Check sheet for the modelled part. Datum: model origin and axes. Units: mm. Face numbers are marked on the shaded views. A direction names the side the tool comes from. Round coordinates to 2 decimals unless told otherwise and drop trailing zeros. Write each loop counter-clockwise with the first axis right and the second up, starting at its lowest first coordinate (ties: lowest second). Pieces come first, ordered by that corner, then holes. Notation, with made-up numbers: (11.5, 57) -> (59.5, 57) arc R7 ccw to (59.5, 70) -> close; hole circle Ø11 at (-37, -0.5). An arc over 180 degrees is marked (long way). One line per item, written item: value.
from build123d import *

# Parameters (mm, degrees)
F0_R     = 1.9
F1_DEPTH = 14.1
F2_DEPTH = 2.1
F3_DEPTH = 10.6
F4_W     = 16.752516
F4_H     = 7.375009
F5_DEPTH = 150
F6_R     = 5
F7_W     = 76.531014
F7_H     = 2.1
F8_DEPTH = 5.5
F9_R     = 1.5


with BuildPart() as f1:
    # F0 (on Top) → F1 (new body)
    with BuildSketch(Plane.XY):
        with BuildLine():
            ThreePointArc((104.3, 0), (101.056497, 1.343503), (102.4, -1.9))
            ThreePointArc((102.4, -1.9), (103.743503, -1.343503), (104.3, 0))
        make_face()
        with BuildLine():
            ThreePointArc((102.4, -23.7), (101.056497, -26.943503), (104.3, -25.6))
            ThreePointArc((104.3, -25.6), (103.743503, -24.256497), (102.4, -23.7))
        make_face()
        with Locations((0, -25.6)):
            Circle(F0_R)
        Circle(F0_R)
    extrude(amount=F1_DEPTH)



with BuildPart() as f2:
    # F0 (on Top) → F2 (new body)
    with BuildSketch(Plane.XY):
        with BuildLine():
            Line((9.95, -14.3), (9.95, -19.3))
            ThreePointArc((9.95, -19.3), (11.414466, -15.764466), (14.95, -14.3))
            Line((14.95, -14.3), (51.2, -14.3))
            Line((51.2, -14.3), (51.2, -11.3))
            Line((51.2, -11.3), (14.95, -11.3))
            ThreePointArc((14.95, -11.3), (11.414466, -9.835534), (9.95, -6.3))
            Line((9.95, -6.3), (9.95, -11.3))
            Line((9.95, -11.3), (9.95, -14.3))
        make_face()
        with BuildLine():
            Line((51.2, -11.3), (51.2, -14.3))
            Line((51.2, -14.3), (67.3, -14.3))
            Line((67.3, -14.3), (72.3, -14.3))
            Line((72.3, -14.3), (87.45, -14.3))
            ThreePointArc((87.45, -14.3), (90.985534, -15.764466), (92.45, -19.3))
            Line((92.45, -19.3), (92.45, -6.3))
            ThreePointArc((92.45, -6.3), (90.985534, -9.835534), (87.45, -11.3))
            Line((87.45, -11.3), (72.3, -11.3))
            Line((72.3, -11.3), (67.3, -11.3))
            Line((67.3, -11.3), (51.2, -11.3))
        make_face()
    extrude(amount=F2_DEPTH)


with BuildPart() as f1_1:
    add(f1.part)

    add(f2.part)  # F3 merges F2
    # F0 (on Top) → F3 (join)
    with BuildSketch(Plane.XY):
        Polygon((-4.5, -30.3), (4.5, -30.3), (4.579243, -30.3), (9.95, -30.3), (9.95, -19.3), (9.95, -14.3), (9.95, -11.3), (9.95, -6.3), (9.95, 4.7), (4.579243, 4.7), (4.5, 4.7), (-4.5, 4.7), align=None)
        with Locations((0, -25.6)):
            Circle(F0_R, mode=Mode.SUBTRACT)
        Circle(F0_R, mode=Mode.SUBTRACT)
        Polygon((92.45, -6.3), (92.45, -19.3), (92.45, -30.3), (97.820757, -30.3), (106.979243, -30.3), (106.979243, 4.7), (97.820757, 4.7), (92.45, 4.7), align=None)
        with BuildLine():
            ThreePointArc((102.4, -23.7), (103.743503, -24.256497), (104.3, -25.6))
            ThreePointArc((104.3, -25.6), (101.056497, -26.943503), (102.4, -23.7))
        make_face(mode=Mode.SUBTRACT)
        with BuildLine():
            ThreePointArc((104.3, 0), (103.743503, -1.343503), (102.4, -1.9))
            ThreePointArc((102.4, -1.9), (101.056497, 1.343503), (104.3, 0))
        make_face(mode=Mode.SUBTRACT)
    extrude(amount=F3_DEPTH)

    # F4 (on Right) → F5 (cut, symmetric)
    with BuildSketch(Plane.YZ):
        with Locations((-12.796251, 8.42476)):
            Rectangle(F4_W, F4_H)
    extrude(amount=F5_DEPTH, both=True, mode=Mode.SUBTRACT)

    # F6
    f6_edges = [f1_1.edges().sort_by_distance(p)[0] for p in [
        (-4.5, 4.7, 5.3),
        (-4.5, -30.3, 5.3),
        (106.979243, 4.7, 5.3),
        (106.979243, -30.3, 5.3),
    ]]
    fillet(f6_edges, radius=F6_R)

    # F7 (on Top) → F8 (join)
    with BuildSketch(Plane.XY):
        Polygon((9.934493, 4.12971), (9.934493, 4.738468), (9.934493, 14.546), (12.934493, 14.546), (12.934493, 16.646), (7.834493, 16.646), (7.834493, 9.642234), (7.834493, 4.738468), (7.834493, 4.12971), align=None)
        with Locations((51.2, 15.596)):
            Rectangle(F7_W, F7_H)
        Polygon((89.465507, 16.646), (89.465507, 14.546), (92.465507, 14.546), (92.465507, 4.738468), (92.465507, 4.379703), (94.565507, 4.379703), (94.565507, 4.738468), (94.565507, 9.642234), (94.565507, 16.646), align=None)
        with Locations((51.2, -41.303271)):
            Rectangle(F7_W, F7_H)
        Polygon((12.934493, -42.353271), (12.934493, -40.253271), (9.934493, -40.253271), (9.934493, -30.445739), (9.934493, -29.831897), (7.834493, -29.831897), (7.834493, -30.445739), (7.834493, -35.349505), (7.834493, -42.353271), align=None)
        Polygon((92.465507, -40.253271), (89.465507, -40.253271), (89.465507, -42.353271), (94.565507, -42.353271), (94.565507, -35.349505), (94.565507, -30.445739), (94.565507, -29.955346), (92.465507, -29.955346), (92.465507, -30.445739), align=None)
    extrude(amount=F8_DEPTH)

    # F9
    f9_edges = [f1_1.edges().sort_by_distance(p)[0] for p in [
        (94.565507, -42.353271, 2.75),
        (94.565507, 16.646, 2.75),
        (7.834493, 16.646, 2.75),
        (7.834493, -42.353271, 2.75),
    ]]
    fillet(f9_edges, radius=F9_R)


solid = f1_1.part
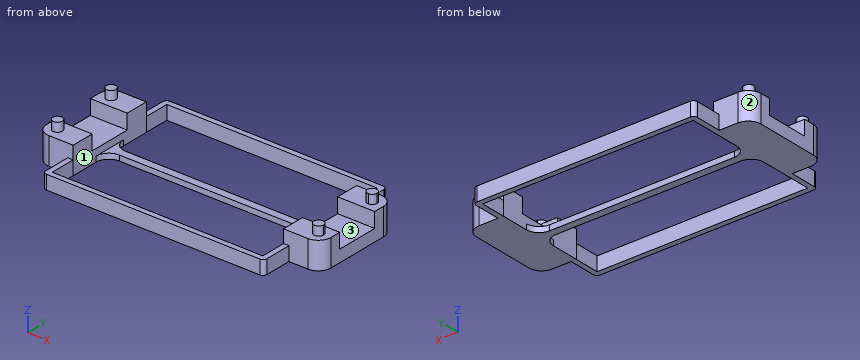
Item 1: Material ranges on line 1 along X through (y, z) = (-39, 0.5); line 2 along X through (y, z) = (-12, 4.5); line 3 along Y through (x, z) = (25, 3.5), recorded low to high.
Result set:
line 1: 7.83 to 9.93, 92.47 to 94.57
line 2: -4.5 to 9.95, 92.45 to 106.98
line 3: -42.35 to -40.25, 14.55 to 16.65
Item 2: Sectioned sample at A-A (y = 7.5). Enter the section's corners in (x, z).
Result set:
outline: (7.83, 0) -> (9.93, 0) -> (9.93, 5.5) -> (7.83, 5.5) -> close; (92.47, 0) -> (94.57, 0) -> (94.57, 5.5) -> (92.47, 5.5) -> close
Item 3: Depth check by flat-ended pin: pin 1 (1.6 mm diameter, centred on y = -37, z = 3.5, fed in from +X); pin 2 (3 mm diameter, centred on y = -27, z = 8.5, fed in from +X); pin 3 (9.5 mm diameter, centred on x = 72.5, y = 11.5, fed in from +Z). Enter the tip coordinate at first touch or a pass-through.
Result set:
pin 1: x = 94.57
pin 2: x = 106.98
pin 3: z = 5.5
Item 4: Tool access check on the marked faces 1, 2 and 3. Record the directions out of +Z, -Z, +X, -X, +Y, -Y that give a thin tool (end or side, any length) a straight path to the whole face; none if there is none.
Result set:
face 1: +Z
face 2: +Z, -Z, -X, +Y
face 3: +Z, +X, -X
Item 5: Sectioned sample at B-B (x = 65). Enter the section's corners in (y, z).
Result set:
outline: (-42.35, 0) -> (-40.25, 0) -> (-40.25, 5.5) -> (-42.35, 5.5) -> close; (-14.3, 0) -> (-11.3, 0) -> (-11.3, 2.1) -> (-14.3, 2.1) -> close; (14.55, 0) -> (16.65, 0) -> (16.65, 5.5) -> (14.55, 5.5) -> close
Item 6: Sectioned sample at D-D (x = 89). Enter the section's corners in (y, z), then the cut area to 3 significant figures.
Result set:
outline: (-42.35, 0) -> (-40.25, 0) -> (-40.25, 5.5) -> (-42.35, 5.5) -> close; (-14.55, 0) -> (-11.05, 0) -> (-11.05, 2.1) -> (-14.55, 2.1) -> close; (14.55, 0) -> (16.65, 0) -> (16.65, 5.5) -> (14.55, 5.5) -> close
area: 30.4 mm^2
Item 7: Sectioned sample at C-C (y = -22.5). Enter the section's corners in (x, z), then the cut area to 3 significant figures.
Result set:
outline: (-4.5, 0) -> (9.95, 0) -> (9.95, 10.6) -> (-4.5, 10.6) -> close; (92.45, 0) -> (106.98, 0) -> (106.98, 10.6) -> (92.45, 10.6) -> close
area: 307 mm^2
